The listing builds one solid part. Answer for the finished solid, in the listing's coordinates (mm). Face numbers are marked on the shaded views. Coordinates: 2 decimals unless noted, no trailing zeros. Order: outer loops, then holes, each group sorted by start corner. A loop starts at its lowest first (then second) coordinate and runs counter-clockwise, first axis right, second up.
```python
from build123d import *

# Parameters (mm, degrees)
SKETCH1_W           = 16
SKETCH1_H           = 4
BOSS_EXTRUDE1_DEPTH = 25
SKETCH2_W           = 16
SKETCH2_H           = 35
BOSS_EXTRUDE2_DEPTH = 2
FILLET1_R           = 3
SKETCH9_W           = 16
SKETCH9_H           = 5.5
CUT_EXTRUDE6_DEPTH  = 10
SKETCH10_W          = 16
SKETCH10_H          = 2
BOSS_EXTRUDE4_DEPTH = 8
SKETCH12_R          = 1.5
CUT_EXTRUDE7_DEPTH  = 10
SKETCH13_R          = 1
CUT_EXTRUDE8_DEPTH  = 10
BOSS_EXTRUDE5_START = 17
BOSS_EXTRUDE5_DEPTH = 17
SKETCH15_W          = 33
SKETCH15_H          = 1.5
CUT_EXTRUDE9_DEPTH  = 10
SKETCH17_W          = 7.5
SKETCH17_H          = 25
CUT_EXTRUDE11_DEPTH = 10
SKETCH18_R          = 1.1
CUT_EXTRUDE12_DEPTH = 27
SKETCH19_W          = 2
SKETCH19_H          = 35
CUT_EXTRUDE13_DEPTH = 27
SKETCH21_W          = 2
SKETCH21_H          = 25
BOSS_EXTRUDE6_DEPTH = 2
SKETCH22_R          = 1.5
CUT_EXTRUDE14_DEPTH = 11
FILLET2_R           = 1
SKETCH23_R          = 1.25
CUT_EXTRUDE15_DEPTH = 10


with BuildPart() as part:
    # Sketch1 → Boss-Extrude1 (new body)
    with BuildSketch(Plane.XY):
        Rectangle(SKETCH1_W, SKETCH1_H)
    extrude(amount=BOSS_EXTRUDE1_DEPTH)

    # Sketch2 → Boss-Extrude2 (add)
    with BuildSketch(Plane.XY.offset(25)):
        with Locations((0, 15.5)):
            Rectangle(SKETCH2_W, SKETCH2_H)
    extrude(amount=BOSS_EXTRUDE2_DEPTH)

    # Fillet1
    fillet1_edges = [part.edges().sort_by_distance(p)[0] for p in [
        (0, 2, 25),
    ]]
    fillet(fillet1_edges, radius=FILLET1_R)

    # Sketch9 → Cut-Extrude6 (cut)
    with BuildSketch(Plane(origin=(0, 2, 0), x_dir=(1, 0, 0), z_dir=(0, 1, 0))):
        with Locations((0, -2.75)):
            Rectangle(SKETCH9_W, SKETCH9_H)
    extrude(amount=-CUT_EXTRUDE6_DEPTH, mode=Mode.SUBTRACT)

    # Sketch10 → Boss-Extrude4 (add)
    with BuildSketch(Plane(origin=(0, 2, 0), x_dir=(1, 0, 0), z_dir=(0, 1, 0))):
        with Locations((0, -6.5)):
            Rectangle(SKETCH10_W, SKETCH10_H)
    extrude(amount=BOSS_EXTRUDE4_DEPTH)

    # Sketch12 → Cut-Extrude7 (cut)
    with BuildSketch(Plane.XY.offset(7.5)):
        with Locations((5, 5.69348198)):
            Circle(SKETCH12_R)
    extrude(amount=-CUT_EXTRUDE7_DEPTH, mode=Mode.SUBTRACT)

    # Sketch13 → Cut-Extrude8 (cut)
    with BuildSketch(Plane.XY.offset(27)):
        with Locations((4, 27.4)):
            Circle(SKETCH13_R)
        with Locations((4, 11.4)):
            Circle(SKETCH13_R)
    extrude(amount=-CUT_EXTRUDE8_DEPTH, mode=Mode.SUBTRACT)

    # Sketch14 → Boss-Extrude5 (add)
    with BuildSketch(Plane.ZY.offset(8).offset(BOSS_EXTRUDE5_START)):
        with BuildLine():
            Line((5.5, 10), (7.5, 10))
            Line((7.5, 10), (7.5, 2))
            Line((7.5, 2), (22, 2))
            ThreePointArc((22, 2), (24.121320344, 2.878679656), (25, 5))
            Line((25, 5), (25, 33))
            Line((25, 33), (27, 33))
            Line((27, 33), (27, -2))
            Line((27, -2), (5.5, -2))
            Line((5.5, -2), (5.5, 10))
        make_face()
    extrude(amount=-BOSS_EXTRUDE5_DEPTH)

    # Sketch15 → Cut-Extrude9 (cut)
    with BuildSketch(Plane(origin=(0, 0, 5.5), x_dir=(-1, 0, 0), z_dir=(0, 0, -1))):
        with Locations((8.5, 9.25)):
            Rectangle(SKETCH15_W, SKETCH15_H)
    extrude(amount=-CUT_EXTRUDE9_DEPTH, mode=Mode.SUBTRACT)

    # Sketch17 → Cut-Extrude11 (cut)
    with BuildSketch(Plane.XY.offset(27)):
        with Locations((-12.25, 15.5)):
            Rectangle(SKETCH17_W, SKETCH17_H)
        with Locations((-4.75, 15.5)):
            Rectangle(SKETCH17_W, SKETCH17_H)
    extrude(amount=-CUT_EXTRUDE11_DEPTH, mode=Mode.SUBTRACT)

    # Sketch18 → Cut-Extrude12 (cut)
    with BuildSketch(Plane(origin=(0, 0, 25), x_dir=(-1, 0, 0), z_dir=(0, 0, -1))):
        with Locations((19, 11.4)):
            Circle(SKETCH18_R)
        with Locations((19, 27.4)):
            Circle(SKETCH18_R)
        with Locations((-4, 27.4)):
            Circle(SKETCH18_R)
        with Locations((-4, 11.4)):
            Circle(SKETCH18_R)
    extrude(amount=-CUT_EXTRUDE12_DEPTH, mode=Mode.SUBTRACT)

    # Sketch19 → Cut-Extrude13 (cut)
    with BuildSketch(Plane(origin=(0, 0, 5.5), x_dir=(-1, 0, 0), z_dir=(0, 0, -1))):
        with Locations((24, 15.5)):
            Rectangle(SKETCH19_W, SKETCH19_H)
    extrude(amount=-CUT_EXTRUDE13_DEPTH, mode=Mode.SUBTRACT)

    # Sketch21 → Boss-Extrude6 (add)
    with BuildSketch(Plane.XY.offset(27)):
        with Locations((-15, 15.5)):
            Rectangle(SKETCH21_W, SKETCH21_H)
    extrude(amount=-BOSS_EXTRUDE6_DEPTH)

    # Sketch22 → Cut-Extrude14 (cut)
    with BuildSketch(Plane(origin=(0, 0, 5.5), x_dir=(-1, 0, 0), z_dir=(0, 0, -1))):
        with Locations((20, 5.69348198)):
            Circle(SKETCH22_R)
    extrude(amount=-CUT_EXTRUDE14_DEPTH, mode=Mode.SUBTRACT)

    # Fillet2
    fillet2_edges = [part.edges().sort_by_distance(p)[0] for p in [
        (-7.5, 2, 7.5),
    ]]
    fillet(fillet2_edges, radius=FILLET2_R)

    # Sketch23 → Cut-Extrude15 (cut)
    with BuildSketch(Plane.XY.offset(27)):
        with Locations((4, 27.4)):
            Circle(SKETCH23_R)
        with Locations((4, 11.4)):
            Circle(SKETCH23_R)
        with Locations((-19, 11.4)):
            Circle(SKETCH23_R)
        with Locations((-19, 27.4)):
            Circle(SKETCH23_R)
    extrude(amount=-CUT_EXTRUDE15_DEPTH, mode=Mode.SUBTRACT)


solid = part.part
```
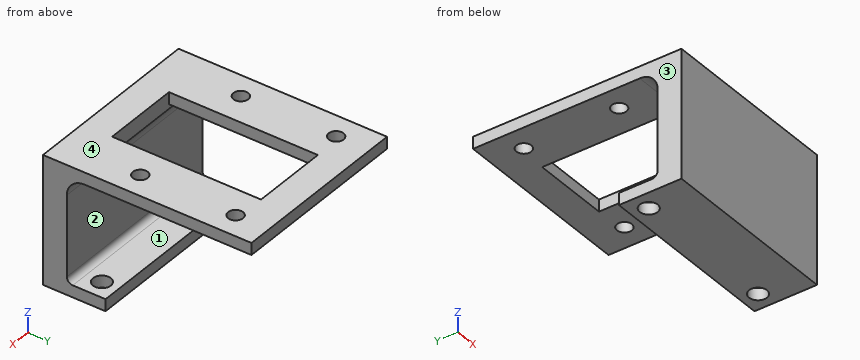
(1) Find section A-A (y = 8). Write down the section's boundary in (x, z), and give its area (3 significant figures).
(2) Find section B-B (x = -6.5). Write down the section's boundary in (y, z), and give its area (3 significant figures).
(3) Find section C-C (y = 27.4). Write down the section's boundary in (x, z), and give its area (3 significant figures).
(4) Consider line 1 (Y direction, x = -19, z = 26.4); line 2 (X direction, y = 25.5, z = 25.5); line 3 (Y direction, x = -20, z = 6.5). Determine where each line is inside the solid, lowest interval first.
(5) The mould has two halves that part along Z. Classify the marked faces 1, 2, 3 and 4: released by +Z, released by -Z, zero draft, split by the parting line, or undercut.
(6) Each of these flat-tipped pins is pushed along its axis until it touches: pin 1 Ø5 at (y, z) = (13, 8) entering from -X; pin 2 Ø4 at (x, y) = (-19, 11.4) entering from -Z; pin 3 Ø2.5 at (x, y) = (-20, 5.69) entering from -Z; pin 4 Ø7 at (x, z) = (-14, 15) entering from +Y. Where does it stop, or does it pass through?
(7) Find section D-D (x = -19). Write down the section's boundary in (y, z), and give its area (3 significant figures).
Findings below:
1. outline: (-23, 5.5) - (8, 5.5) - (8, 7.5) - (-23, 7.5) - close; (-23, 25) - (-14, 25) - (-14, 27) - (-23, 27) - close; (-1, 25) - (8, 25) - (8, 27) - (-1, 27) - close
1. area: 98.0 mm2
2. outline: (-2, 5.5) - (8.5, 5.5) - (8.5, 7.5) - (3, 7.5) arc R1 cw to (2, 8.5) - (2, 22) arc R3 cw to (3, 24.24) - (3, 27) - (-2, 27) - close; (28, 25) - (33, 25) - (33, 27) - (28, 27) - close
2. area: 113 mm2
3. outline: (-23, 25) - (-20.25, 25) - (-20.25, 27) - (-23, 27) - close; (-17.75, 25) - (-14, 25) - (-14, 27) - (-17.75, 27) - close; (-1, 25) - (2.75, 25) - (2.75, 27) - (-1, 27) - close; (5.25, 25) - (8, 25) - (8, 27) - (5.25, 27) - close
3. area: 26.0 mm2
4. line 1: y = -2 to 10.15, 12.65 to 26.15, 28.65 to 33
4. line 2: x = -23 to -14, -1 to 8
4. line 3: y = -2 to 4.19, 7.19 to 8.5
5. face 1: undercut
5. face 2: undercut
5. face 3: zero draft
5. face 4: released by +Z
6. pin 1: passes through
6. pin 2: stops at z = 25
6. pin 3: stops at z = 24.95
6. pin 4: stops at y = 2
7. outline: (-2, 5.5) - (4.58, 5.5) - (4.58, 7.5) - (3, 7.5) arc R1 cw to (2, 8.5) - (2, 22) arc R3 cw to (5, 25) - (10.15, 25) - (10.15, 27) - (-2, 27) - close; (6.81, 5.5) - (8.5, 5.5) - (8.5, 7.5) - (6.81, 7.5) - close; (12.65, 25) - (26.15, 25) - (26.15, 27) - (12.65, 27) - close; (28.65, 25) - (33, 25) - (33, 27) - (28.65, 27) - close
7. area: 149 mm2
